Geometry: final body of the model. Coordinates: model frame, mm. A direction names the side the tool comes from. Give positions to 0.01 mm unless a question says otherwise; leave off trailing zeros. Write each loop counter-clockwise with the first axis right and the second up, starting at its lowest first coordinate (ties: lowest second). Pieces come first, ordered by that corner, then holes. Notation, with made-up numbers: (59, 54) -> (114, 54) arc R30 cw to (114, 79) -> close; hole circle Ø3 at (11.25, -15). An arc over 180 degrees is marked (long way). Answer as a JSON object with one key per item and string values. Group by question number.
(1) Section query C-C on y = 66.5. Output: boundary loops of the cut face in (x, z).
(2) Section query B-B on x = 0. Output: boundary loops of the cut face in (y, z), plus the area to 3 significant figures.
(3) Section query A-A on z = 0. Output: boundary loops of the cut face in (x, y).
(4) Section query D-D on x = -8.5. Output: boundary loops of the cut face in (y, z).
(5) Set-up query: faces 1 (the face through (0, 100.635, 0)), 2 (the face through (3.258, 10.782, -6.264)). Return all of +Z, -Z, +X, -X, +Y, -Y with unobstructed straight access to the full face (end or side cutting, diameter ignored); none if empty.
(6) Material intervals for probe 1 along X at (y, z) = (7.5, -0.25); probe 2 along Y at (x, z) = (-8.5, 5.5); probe 3 along X at (y, z) = (82, -1), sorted ascending.
(7) Contact query for flat-ended pins moving along their axis: pin 1 Ø1 at (y, z) = (42.5, -7.5) entering from -X; pin 2 Ø4 at (x, y) = (0.5, 64) entering from -Z; pin 3 Ø6 at (x, z) = (-8.5, -10.5) entering from -Y; pin 4 Ø10 at (y, z) = (38, 9.5) entering from -X. Output: stop coordinate, or through.
from build123d import *

# Parameters (mm, degrees)
F0_R     = 7.0612
F1_DEPTH = 21.8694
F3_R     = 10.6807
F4_DEPTH = 30.5562
F6_R     = 14.9606
F7_DEPTH = 48.2092


with BuildPart() as f1:
    # F0 (on Front) → F1 (new body)
    with BuildSketch(Plane.XZ):
        Circle(F0_R)
    extrude(amount=-F1_DEPTH)

    # F3 (on offset) → F4 (join)
    with BuildSketch(Plane(origin=(0, 21.8694, 0), x_dir=(1, 0, 0), z_dir=(0, 1, 0))):
        Circle(F3_R)
    extrude(amount=F4_DEPTH)

    # F6 (on offset) → F7 (join)
    with BuildSketch(Plane(origin=(0, 52.4256, 0), x_dir=(1, 0, 0), z_dir=(0, 1, 0))):
        Circle(F6_R)
    extrude(amount=F7_DEPTH)


solid = f1.part
Answer list:
{
 "1": {"outline": "circle Ø29.92 at (0, 0)"},
 "2": {"outline": "(0, -7.06) -> (21.87, -7.06) -> (21.87, -10.68) -> (52.43, -10.68) -> (52.43, -14.96) -> (100.63, -14.96) -> (100.63, 14.96) -> (52.43, 14.96) -> (52.43, 10.68) -> (21.87, 10.68) -> (21.87, 7.06) -> (0, 7.06) -> close", "area": "2,400 mm2"},
 "3": {"outline": "(-14.96, 52.43) -> (-10.68, 52.43) -> (-10.68, 21.87) -> (-7.06, 21.87) -> (-7.06, 0) -> (7.06, 0) -> (7.06, 21.87) -> (10.68, 21.87) -> (10.68, 52.43) -> (14.96, 52.43) -> (14.96, 100.63) -> (-14.96, 100.63) -> close"},
 "4": {"outline": "(21.87, -6.47) -> (52.43, -6.47) -> (52.43, -12.31) -> (100.63, -12.31) -> (100.63, 12.31) -> (52.43, 12.31) -> (52.43, 6.47) -> (21.87, 6.47) -> close"},
 "5": {"face 1": "+Z, -Z, +X, -X, +Y", "face 2": "-Y"},
 "6": {"probe 1": "-7.06 to 7.06", "probe 2": "21.87 to 100.63", "probe 3": "-14.93 to 14.93"},
 "7": {"pin 1": "x = -8.07", "pin 2": "z = -14.96", "pin 3": "y = 21.87", "pin 4": "x = -9.69"}
}
